Input: part model. Units: mm. Frame: model coordinates. Face numbers are marked on the shaded views. Coordinates: 2 decimals unless noted, no trailing zeros. Order: outer loops, then holes, each group sorted by start corner. A loop starts at its lowest first (then second) coordinate and runs counter-clockwise, first axis right, second up. Notation, with made-up numbers: (17, 29.25) -> (73, 29.25) arc R35 cw to (73, 61.25) -> close; hole circle Ø3 at (-22, 87.5). An arc over 180 degrees is marked (long way). Write each question's results on one line, items separated by ' | '.
```python
from build123d import *

# Parameters (mm, degrees)
ESQUISSE1_R             = 35
BOSS_EXTRU_2_DEPTH      = 250
ESQUISSE4_R             = 34
ENL_V_MAT_EXTRU_3_DEPTH = 250
ESQUISSE5_R             = 36
BOSS_EXTRU_5_DEPTH      = 200
ESQUISSE6_R             = 34
ENL_V_MAT_EXTRU_4_DEPTH = 200


with BuildPart() as part:
    # Esquisse1 → Boss.-Extru.2 (new body)
    with BuildSketch(Plane(origin=(0, 0, 0), x_dir=(1, 0, 0), z_dir=(0, 1, 0))):
        with Locations(Location((0, 0, 0), (0, 0, 270))):
            Circle(ESQUISSE1_R)
    extrude(amount=BOSS_EXTRU_2_DEPTH)

    # Esquisse4 → Enlèv. mat.-Extru.3 (cut)
    with BuildSketch(Plane(origin=(0, 250, 0), x_dir=(1, 0, 0), z_dir=(0, 1, 0))):
        with Locations(Location((0, 0, 0), (0, 0, 270))):
            Circle(ESQUISSE4_R)
    extrude(amount=-ENL_V_MAT_EXTRU_3_DEPTH, mode=Mode.SUBTRACT)

    # Esquisse5 → Boss.-Extru.5 (add)
    with BuildSketch(Plane(origin=(0, 250, 0), x_dir=(1, 0, 0), z_dir=(0, 1, 0))):
        with Locations(Location((0, 0, 0), (0, 0, 270))):
            Circle(ESQUISSE5_R)
    extrude(amount=-BOSS_EXTRU_5_DEPTH)

    # Esquisse6 → Enlèv. mat.-Extru.4 (cut)
    with BuildSketch(Plane(origin=(0, 250, 0), x_dir=(1, 0, 0), z_dir=(0, 1, 0))):
        with Locations(Location((0, 0, 0), (0, 0, 270))):
            Circle(ESQUISSE6_R)
    extrude(amount=-ENL_V_MAT_EXTRU_4_DEPTH, mode=Mode.SUBTRACT)


solid = part.part
```
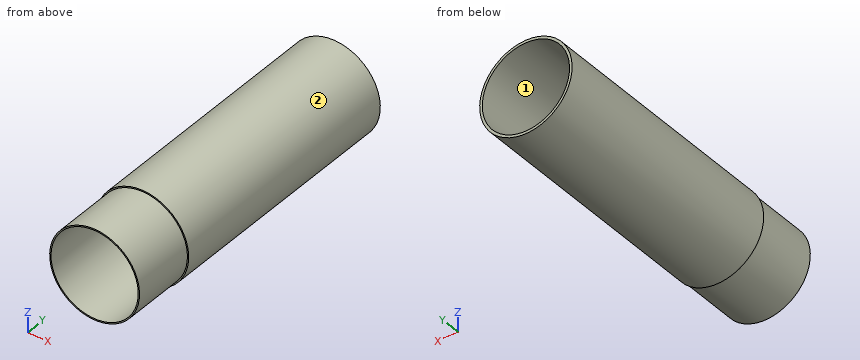
(1) Line query: line 1 along X through (y, z) = (65, 0); line 2 along Z through (x, y) = (29, 166); line 3 along Z through (x, y) = (-11, 34.5). Output: solid intervals per line, ascending. Write a range as from..to.
Return value:
line 1: -36..-34, 34..36 | line 2: -21.33..-17.75, 17.75..21.33 | line 3: -33.23..-32.17, 32.17..33.23
(2) Mould query, pull axis X, two halves, no side actions, for the marked faces 1 and 2. Classes: +X half, -X half, draft (parallel to the pull), parting line (faces both ways), or undercut.
Return value:
face 1: undercut | face 2: parting line
(3) Cut plane A-A, the plane z = 0. Return loops of the section in (x, y), plus the area to 3 significant figures.
Return value:
outline: (-36, 50) -> (-35, 50) -> (-35, 0) -> (-34, 0) -> (-34, 250) -> (-36, 250) -> close; (34, 0) -> (35, 0) -> (35, 50) -> (36, 50) -> (36, 250) -> (34, 250) -> close | area: 900 mm2
(4) Cut plane B-B, the plane x = 15. Return loops of the section in (y, z), plus the area to 3 significant figures.
Return value:
outline: (0, -31.62) -> (50, -31.62) -> (50, -32.73) -> (250, -32.73) -> (250, -30.51) -> (0, -30.51) -> close; (0, 30.51) -> (250, 30.51) -> (250, 32.73) -> (50, 32.73) -> (50, 31.62) -> (0, 31.62) -> close | area: 997 mm2
(5) Cut plane C-C, the plane y = 122. Return loops of the section in (x, z), plus the area to 3 significant figures.
Return value:
outline: circle Ø72 at (0, 0); hole circle Ø68 at (0, 0) | area: 440 mm2
(6) Cut plane D-D, the plane y = 47. Return loops of the section in (x, z).
Return value:
outline: circle Ø70 at (0, 0); hole circle Ø68 at (0, 0)
(7) Pin query (flat end, axial travel): P1, Ø4, axis at x = -24.5, z = 28, coming from the -Y side; P2, Ø10, axis at x = 25.5, y = 138, coming from the -Z side; P3, Ø1, axis at x = -15, y = 195.5, coming from the +Z side. Return the tip coordinate at first contact, or that it passes through.
Return value:
P1: y = 50 | P2: z = -29.59 | P3: z = 32.95
